Here's how the part is built. I have some questions about the finished solid (model axes, mm). Face numbers are marked on the shaded views. Round coordinates to 2 decimals unless told otherwise and drop trailing zeros. Loops run counter-clockwise (first coordinate to the right, second up) from the corner with the lowest first, then second, coordinate; pieces in that order, holes last. Notation, with made-up numbers: M -34,82.5 L -16,82.5 A27 ccw -16,103.5 Z; hole C -18.75,77 d6. An arc over 180 degrees is marked long. Answer as a JSON object with one key per item and string values.
Autodesk Fusion 360 part; units mm, degrees
sketch "Boceto1" plane through (0, 0, 0) normal (0, 0, 1) x (1, 0, 0)
  line L0 (15, 15) -> (-15, 15)
  line L1 (-15, 15) -> (-15, -15)
  line L2 (-15, -15) -> (15, -15)
  line L3 (15, -15) -> (15, 15)
  line L4 (15, 15) -> (-15, -15) construction
  line L5 (-15, 15) -> (15, -15) construction
  line L6 (12.5, 12.5) -> (-12.5, 12.5)
  line L7 (-12.5, 12.5) -> (-12.5, -12.5)
  line L8 (-12.5, -12.5) -> (12.5, -12.5)
  line L9 (12.5, -12.5) -> (12.5, 12.5)
  line L10 (12.5, 12.5) -> (-12.5, -12.5) construction
  line L11 (-12.5, 12.5) -> (12.5, -12.5) construction
  line L12 (11, -11) -> (-11, -11)
  line L13 (-11, -11) -> (-11, 11)
  line L14 (-11, 11) -> (11, 11)
  line L15 (11, 11) -> (11, -11)
  line L16 (11, -11) -> (-11, 11) construction
  line L17 (-11, -11) -> (11, 11) construction
  dimension "d1" = 30
  dimension "d2" = 30
  dimension "d3" = 25
  dimension "d4" = 25
  dimension "d7" = 22
  dimension "d8" = 22
extrude "Extruir1" add sketch "Boceto1" along normal blind 3 contours L0 L1 L2 L3 | L6 L7 L8 L9 | L12 L13 L14 L15 makes body 1
extrude "Extruir2" add sketch "Boceto1" against normal blind 2 separate body contours L6 L7 L8 L9 makes body 2
combine "Combinar1" operation add target body 2 tool bodies 1
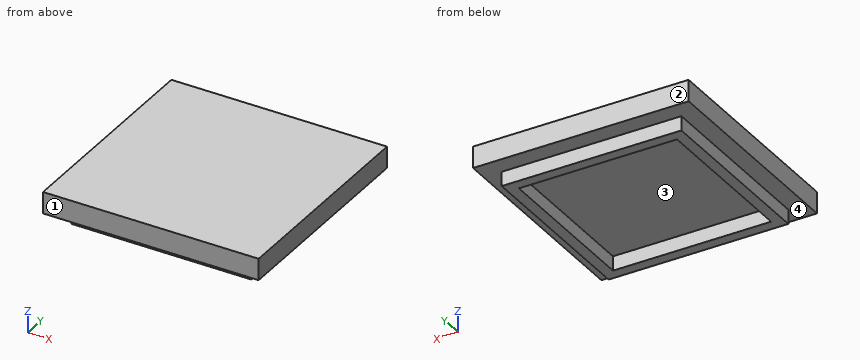
Item 1: I want a section at D-D on x = -11.75. List the corners of the cut face in (y, z) for me.
Solution:
{"outline": "M -15,0 L -12.5,0 L -12.5,-2 L 12.5,-2 L 12.5,0 L 15,0 L 15,3 L -15,3 Z"}
Item 2: I want a section at B-B on x = -0.25. List the corners of the cut face in (y, z) for me.
Solution:
{"outline": "M -15,0 L -12.5,0 L -12.5,-2 L -11,-2 L -11,0 L 11,0 L 11,-2 L 12.5,-2 L 12.5,0 L 15,0 L 15,3 L -15,3 Z"}
Item 3: We'd pull the mould along Y, two halves only. Please class the marked faces 1, 2, 3 and 4: +Y half, -Y half, draft (parallel to the pull), parting line (faces both ways), or undercut.
Solution:
{"face 1": "-Y half", "face 2": "+Y half", "face 3": "undercut", "face 4": "draft"}
Item 4: I want a section at A-A on z = -1.65. List the corners of the cut face in (x, y) for me, plus the area to 3 significant figures.
Solution:
{"outline": "M -12.5,-12.5 L 12.5,-12.5 L 12.5,12.5 L -12.5,12.5 Z; hole M -11,-11 L 11,-11 L 11,11 L -11,11 Z", "area": "141 mm2"}
Item 5: If I drill on L1, parallel to X at y = 4.25, z = -0.3; L2, parallel to Z at x = 3, y = 2.5, over which ranges is the centre line in solid material (lowest first)? Write a range as from..to.
Solution:
{"L1": "x = -12.5..-11, 11..12.5", "L2": "z = 0..3"}
Item 6: For P1, Ø2, axis at x = -4.5, z = -1.5, coming from the -Y side; P2, Ø1.5, axis at x = -7.5, z = -0.5, coming from the -Y side; P3, Ø3, axis at x = 5, y = 1, coming from the -Z side; P4, Ø0.6, axis at x = 3.5, z = -1, coming from the +Y side, each with a flat end and sliding along its axis, tell me the tip position at first contact or that it passes through.
Solution:
{"P1": "stops at y = -12.5", "P2": "stops at y = -15", "P3": "stops at z = 0", "P4": "stops at y = 12.5"}
